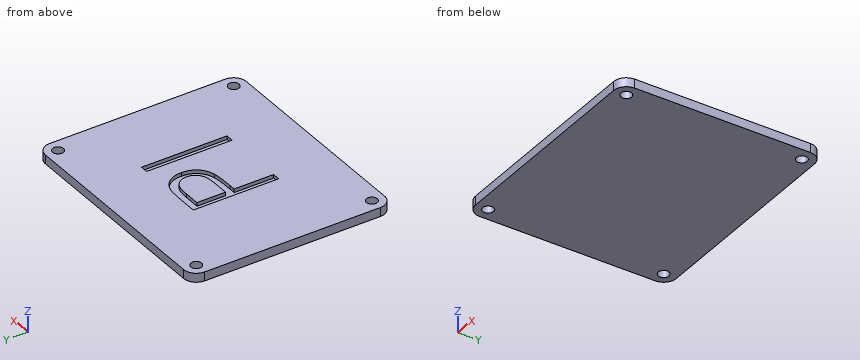
```python
from build123d import *

# Parameters (mm, degrees)
BOSS_EXTRU_1_OUTLINE_W  = 65
BOSS_EXTRU_1_OUTLINE_H  = 56
BOSS_EXTRU_1_OUTLINE_R  = 1.5
BOSS_EXTRU_1_DEPTH      = 2.5
CONG_3_R                = 3.5
ESQUISSE2_W             = 2.137019231
ESQUISSE2_H             = 23.8125
ENL_V_MAT_EXTRU_1_DEPTH = 1


# Read off the part's stored shape, not the designer's step: Boss.-Extru.1
with BuildPart() as part:
    # Boss.-Extru.1 outline → Boss.-Extru.1 (new body)
    with BuildSketch(Plane.XY):
        Rectangle(BOSS_EXTRU_1_OUTLINE_W, BOSS_EXTRU_1_OUTLINE_H)
        with Locations((-29, -24.5)):
            Circle(BOSS_EXTRU_1_OUTLINE_R, mode=Mode.SUBTRACT)
        with Locations((29, -24.5)):
            Circle(BOSS_EXTRU_1_OUTLINE_R, mode=Mode.SUBTRACT)
        with Locations((-29, 24.5)):
            Circle(BOSS_EXTRU_1_OUTLINE_R, mode=Mode.SUBTRACT)
        with Locations((29, 24.5)):
            Circle(BOSS_EXTRU_1_OUTLINE_R, mode=Mode.SUBTRACT)
    extrude(amount=BOSS_EXTRU_1_DEPTH)

    # Congé3
    cong_3_edges = [part.edges().sort_by_distance(p)[0] for p in [
        (-32.5, 28, 1.25),
        (32.5, 28, 1.25),
        (32.5, -28, 1.25),
        (-32.5, -28, 1.25),
    ]]
    fillet(cong_3_edges, radius=CONG_3_R)

    # Esquisse2 → Enlèv. mat.-Extru.1 (cut)
    # profile 1 of 2: a face of its own
    with BuildSketch(Plane.XY.offset(2.5)):
        with BuildLine():
            Line((-9.322744099, 12.249768252), (-4.652784664, 12.249768252))
            add(Edge.make_bspline(
                [(-4.652784664, 12.249768252), (-4.331581892, 12.249415172), (-3.716143116, 12.248738655), (-2.833617469, 12.228227617), (-2.032090545, 12.20083173), (-1.313290632, 12.16285492), (-0.675006107, 12.117974548), (-0.120125194, 12.055027637), (0.355713573, 11.989303126), (0.640827095, 11.922482485), (0.77085566, 11.892008336)],
                knots=[0, 0, 0, 0, 1.415646017, 2.712440637, 3.8905458, 4.950247383, 5.884950622, 6.709939814, 7.411656543, 8, 8, 8, 8], degree=3))
            add(Edge.make_bspline(
                [(0.77085566, 11.892008336), (0.935458095, 11.846955427), (1.260784315, 11.757911225), (1.729557484, 11.579564285), (2.175557754, 11.368094554), (2.600315321, 11.127085249), (2.998610565, 10.846195964), (3.376385951, 10.536812958), (3.730307602, 10.191793179), (4.058385286, 9.815006359), (4.35968007, 9.412777789), (4.61909809, 8.979102974), (4.83631726, 8.521281785), (5.022621303, 8.039632667), (5.156709181, 7.530111002), (5.257721123, 6.996257119), (5.321835447, 6.438128245), (5.32797609, 6.056720932), (5.331102055, 5.86256122)],
                knots=[0, 0, 0, 0, 0.999701418, 1.975846123, 2.934577507, 3.890451536, 4.834027766, 5.787354733, 6.749476667, 7.726910423, 8.712836071, 9.690891519, 10.682875813, 11.679750201, 12.712814741, 13.765529915, 14.8625177, 16, 16, 16, 16], degree=3))
            add(Edge.make_bspline(
                [(5.331102055, 5.86256122), (5.328234861, 5.66676956), (5.322625004, 5.283689954), (5.25529492, 4.723260806), (5.164602009, 4.187694616), (5.025148849, 3.67817889), (4.842502395, 3.197739452), (4.628243964, 2.739034284), (4.369820302, 2.309867231), (4.072879586, 1.908680234), (3.742555345, 1.535096724), (3.380245177, 1.191823926), (2.987411776, 0.880871195), (2.56530359, 0.601541428), (2.109805511, 0.360312098), (1.627825859, 0.144249005), (1.11517528, -0.037209461), (0.760419961, -0.132663986), (0.580050372, -0.181196292)],
                knots=[0, 0, 0, 0, 1.121902311, 2.195077645, 3.232258892, 4.234102512, 5.217864754, 6.176164875, 7.132989551, 8.084763148, 9.034132444, 9.988522005, 10.94243251, 11.903244335, 12.886203696, 13.894208494, 14.929344452, 16, 16, 16, 16], degree=3))
            add(Edge.make_bspline(
                [(0.580050372, -0.181196292), (0.430866189, -0.212921216), (0.103920378, -0.282448234), (-0.434532786, -0.360066485), (-1.061450501, -0.426316947), (-1.775977084, -0.475990758), (-2.577471169, -0.518515586), (-3.466366331, -0.552316368), (-4.444407463, -0.570889123), (-5.126610034, -0.571847017), (-5.482787669, -0.572347133)],
                knots=[0, 0, 0, 0, 0.601384939, 1.31797006, 2.144135048, 3.087295005, 4.142315834, 5.309527816, 6.595305764, 8, 8, 8, 8], degree=3))
            Line((-5.482787669, -0.572347133), (-7.185724869, -0.572347133))
            Line((-7.185724869, -0.572347133), (-7.185724869, -11.562731748))
            Line((-7.185724869, -11.562731748), (-9.322744099, -11.562731748))
            Line((-9.322744099, -11.562731748), (-9.322744099, 12.249768252))
        make_face()
        with BuildLine():
            Line((-7.185724869, 9.807460559), (-7.185724869, 1.869960559))
            Line((-7.185724869, 1.869960559), (-3.016629316, 1.817489105))
            add(Edge.make_bspline(
                [(-3.016629316, 1.817489105), (-2.813066963, 1.817383897), (-2.420094039, 1.817180796), (-1.852429734, 1.844294549), (-1.325770119, 1.875594601), (-0.841732919, 1.921422938), (-0.400099936, 1.986201493), (-0.000134784, 2.051595639), (0.355061194, 2.146201766), (0.770753978, 2.273585505), (1.233963895, 2.490841336), (1.737887752, 2.806186124), (2.16495192, 3.208145942), (2.534510332, 3.660092437), (2.827784252, 4.162870443), (3.042477699, 4.700821602), (3.168623788, 5.268428935), (3.185538784, 5.656832166), (3.194082824, 5.853020956)],
                knots=[0, 0, 0, 0, 1.160613943, 2.240541288, 3.23993089, 4.169200891, 5.011653406, 5.7853311, 6.478053781, 7.106038997, 8.262395093, 9.384106736, 10.481365981, 11.59014053, 12.70357646, 13.786202915, 14.881775077, 16, 16, 16, 16], degree=3))
            add(Edge.make_bspline(
                [(3.194082824, 5.853020956), (3.185492318, 6.044463342), (3.168415456, 6.425027112), (3.041488959, 6.982775465), (2.828201662, 7.515057668), (2.532541618, 8.011535267), (2.173713573, 8.461855522), (1.756659113, 8.853041333), (1.28235996, 9.167513989), (0.841160389, 9.370486852), (0.449266605, 9.49441578), (0.108870592, 9.581126212), (-0.275467747, 9.650356676), (-0.703873532, 9.706414722), (-1.173026277, 9.754403449), (-1.686956598, 9.786965187), (-2.243717635, 9.806025094), (-2.630232412, 9.806970487), (-2.830594159, 9.807460559)],
                knots=[0, 0, 0, 0, 1.120700087, 2.227813068, 3.331159281, 4.466773991, 5.599788987, 6.693661531, 7.80175334, 8.91857717, 9.525282508, 10.207424825, 10.974604443, 11.810962634, 12.737642355, 13.736264703, 14.826523623, 16, 16, 16, 16], degree=3))
            Line((-2.830594159, 9.807460559), (-7.185724869, 9.807460559))
        make_face(mode=Mode.SUBTRACT)
    # profile 2 of 2: a face of its own
    with BuildSketch(Plane.XY.offset(2.5)):
        with Locations((11.284227055, 0.343518252)):
            Rectangle(ESQUISSE2_W, ESQUISSE2_H)
    extrude(amount=-ENL_V_MAT_EXTRU_1_DEPTH, mode=Mode.SUBTRACT)


solid = part.part
```
The model under review builds one solid part; all positions refer to its coordinate system, in mm. Round coordinates to 2 decimals unless told otherwise and drop trailing zeros. Loops run counter-clockwise (first coordinate to the right, second up) from the corner with the lowest first, then second, coordinate; pieces in that order, holes last. Notation, with made-up numbers: (6.5, 38.25) -> (38.5, 38.25) arc R20 cw to (38.5, 74.25) -> close; hole circle Ø1 at (25.5, -16). An arc over 180 degrees is marked (long way). Answer in a Markdown table with one row per item.
1) Wall thickness on line 1 along Y through (x, z) = (-29, 1.9); line 2 along X through (y, z) = (-5.5, 2.2); line 3 along Z through (x, y) = (10.5, 3.5): over which ranges is each line inside the solid? List them lowest first.
Taken from the geometry:
| item | result |
|---|---|
| line 1 | y = -28 to -26, -23 to 23, 26 to 28 |
| line 2 | x = -32.5 to -9.32, -7.19 to 10.22, 12.35 to 32.5 |
| line 3 | z = 0 to 1.5 |
2) Consider section A-A, the plane z = 2. Count the separate pieces of the cut face and the enclosed holes in it, plus the area to 3 significant figures.
Taken from the geometry:
| item | result |
|---|---|
| separate pieces | 2 |
| enclosed holes | 6 |
| area | 3,430 mm² |
3) Consider section B-B, the plane y = -2. Write out the cut boundary in (x, z), plus the area to 3 significant figures.
Taken from the geometry:
| item | result |
|---|---|
| outline | (-32.5, 0) -> (32.5, 0) -> (32.5, 2.5) -> (12.35, 2.5) -> (12.35, 1.5) -> (10.22, 1.5) -> (10.22, 2.5) -> (-7.19, 2.5) -> (-7.19, 1.5) -> (-9.32, 1.5) -> (-9.32, 2.5) -> (-32.5, 2.5) -> close |
| area | 158 mm² |
